Check sheet for the modelled part. Datum: model origin and axes. Units: mm. A direction names the side the tool comes from. Give positions to 0.01 mm unless a question says otherwise; leave off trailing zeros. Write each loop counter-clockwise with the first axis right and the second up, starting at its lowest first coordinate (ties: lowest second). Pieces come first, ordered by that corner, then holes. Notation, with made-up numbers: (22, 85.25) -> (38, 85.25) arc R22 cw to (38, 116.25) -> close; hole circle Ø3 at (60.5, -7.5). An arc over 180 degrees is marked (long way). Use a Markdown table: item, result. Add a question column.
1. Cross-section at B-B (x = 12.2). Enter the section's corners in (y, z).
2. Cross-section at D-D (y = 10.25). Enter the section's corners in (x, z).
3. Release check for a two-part mould opening along X. For faces 5 (the cylindrical face through (14.7, 5.8, 24.7)), 6 (the cylindrical face through (4.075, 4.5, 28.278)), 7 (the flat face through (11, 6, 0)) record: released by +X, released by -X, zero draft, split by the parting line, or undercut.
4. Cross-section at C-C (y = 3). Enter the section's corners in (x, z).
5. Cross-section at A-A (x = -2.4). Enter the section's corners in (y, z), then the cut area to 3 significant figures.
6. Scan lines: probe 1 along Y at (x, z) = (5.9, 27.35); probe 2 along Y at (x, z) = (-2.4, 16.65); probe 3 along X at (y, z) = (5.9, 17.4). Record each from-to range of solid material in increasing order. Write a range as [from, to].
7. Set-up check for faces 1 (the flat face through (22.5, 6, 21)), 2 (the flat face through (0, 6, 8)), 3 (the flat face through (24.8, 7.3, 15.9)), 4 (the cylindrical face through (0, 6, 25)): record each of +Z, -Z, +X, -X, +Y, -Y from which the full face is reachable in a straight line by a thin tool's end or side.
8. Gauge pin test, flat ends, axial feed: P1, Ø2, axis at y = 6.5, z = 20, coming from the +X side; P2, Ø1.8, axis at x = 3, y = 7.5, coming from the +Z side; P3, Ø1.4, axis at x = -1.5, y = 5, coming from the +Z side. Record the tip position at first contact, or that the pin passes through.
from build123d import *

# Parameters (mm, degrees)
CYLINDER005_R             = 0.85
CYLINDER005_DEPTH         = 4
CYLINDER004_R             = 2.3
CYLINDER004_DEPTH         = 3.3
CYLINDER003_R             = 2.5
CYLINDER003_DEPTH         = 4
CYLINDER002_R             = 5.9
CYLINDER002_DEPTH         = 4
BOX003_W                  = 22.5
BOX003_H                  = 11.8
BOX003_DEPTH              = 22.7
BOX002_W                  = 4.3
BOX002_H                  = 1.3
BOX002_DEPTH              = 5
CYLINDER001_R             = 1
CYLINDER001_DEPTH         = 5
FUSION001_PLACEMENT_ANGLE = 180
BOX001_W                  = 4.3
BOX001_H                  = 1.3
BOX001_DEPTH              = 5
CYLINDER_R                = 1
CYLINDER_DEPTH            = 5
BOX_W                     = 31.9
BOX_H                     = 11.8
BOX_DEPTH                 = 2.5


with BuildPart() as cylinder005:
    # Cylinder005 → Cylinder005 (new body)
    with BuildSketch(Plane.XY.offset(-0.5)):
        Circle(CYLINDER005_R)
    extrude(amount=CYLINDER005_DEPTH)


with BuildPart() as rotor:
    # Cylinder004 → Cylinder004 (new body)
    with BuildSketch(Plane.XY.offset(-0.1)):
        Circle(CYLINDER004_R)
    extrude(amount=CYLINDER004_DEPTH)

    # Cut002: cut Cylinder005
    add(cylinder005.part, mode=Mode.SUBTRACT)


with BuildPart() as rotor_1:
    # Cut002 placement: moved
    add(rotor.part.moved(Location((5.9, 5.9, 26.7))))


with BuildPart() as cylinder003:
    # Cylinder003 → Cylinder003 (new body)
    with BuildSketch(Plane(origin=(6.3, 0, 0), x_dir=(1, 0, 0), z_dir=(0, 0, 1))):
        Circle(CYLINDER003_R)
    extrude(amount=CYLINDER003_DEPTH)


with BuildPart() as soporte_con_rotor:
    # Cylinder002 → Cylinder002 (new body)
    with BuildSketch(Plane.XY):
        Circle(CYLINDER002_R)
    extrude(amount=CYLINDER002_DEPTH)

    # Fusion002: union Cylinder003
    add(cylinder003.part)


with BuildPart() as soporte_con_rotor_1:
    # Fusion002 placement: moved
    add(soporte_con_rotor.part.moved(Location((5.9, 5.9, 22.7))))

    # Fusion004: union rotor
    add(rotor_1.part)


with BuildPart() as base:
    # Box003 → Box003 (new body)
    with BuildSketch(Plane.XY):
        with Locations((11.25, 5.9)):
            Rectangle(BOX003_W, BOX003_H)
    extrude(amount=BOX003_DEPTH)


with BuildPart() as taladro_cubo001:
    # Box002 → Box002 (new body)
    with BuildSketch(Plane(origin=(0, -0.65, 0), x_dir=(1, 0, 0), z_dir=(0, 0, 1))):
        with Locations((2.15, 0.65)):
            Rectangle(BOX002_W, BOX002_H)
    extrude(amount=BOX002_DEPTH)


with BuildPart() as fusion001:
    # Cylinder001 → Cylinder001 (new body)
    with BuildSketch(Plane.XY):
        Circle(CYLINDER001_R)
    extrude(amount=CYLINDER001_DEPTH)

    # Fusion001: union taladro-cubo001
    add(taladro_cubo001.part)


with BuildPart() as fusion001_1:
    # Fusion001 placement: moved
    add(fusion001.part.moved(Location((2.3, 5.9, -1))).rotate(Axis((2.3, 5.9, -1), (0, 0, 1)), FUSION001_PLACEMENT_ANGLE))


with BuildPart() as taladro_cubo:
    # Box001 → Box001 (new body)
    with BuildSketch(Plane(origin=(0, -0.65, 0), x_dir=(1, 0, 0), z_dir=(0, 0, 1))):
        with Locations((2.15, 0.65)):
            Rectangle(BOX001_W, BOX001_H)
    extrude(amount=BOX001_DEPTH)


with BuildPart() as fusion:
    # Cylinder → Cylinder (new body)
    with BuildSketch(Plane.XY):
        Circle(CYLINDER_R)
    extrude(amount=CYLINDER_DEPTH)

    # Fusion: union taladro-cubo
    add(taladro_cubo.part)


with BuildPart() as fusion_1:
    # Fusion placement: moved
    add(fusion.part.moved(Location((29.6, 5.9, -1))))


with BuildPart() as fusion005:
    # Box → Box (new body)
    with BuildSketch(Plane.XY):
        with Locations((15.95, 5.9)):
            Rectangle(BOX_W, BOX_H)
    extrude(amount=BOX_DEPTH)

    # Cut: cut Fusion
    add(fusion_1.part, mode=Mode.SUBTRACT)

    # Cut001: cut Fusion001
    add(fusion001_1.part, mode=Mode.SUBTRACT)


with BuildPart() as fusion005_1:
    # Cut001 placement: moved
    add(fusion005.part.moved(Location((-4.7, 0, 15.9))))

    # Fusion003: union base
    add(base.part)

    # Fusion005: union soporte-con-rotor
    add(soporte_con_rotor_1.part)


solid = fusion005_1.part
Worked answers:
| question | item | result |
|---|---|---|
| 1 | outline | (0, 0) -> (11.8, 0) -> (11.8, 22.7) -> (8.4, 22.7) -> (8.4, 26.7) -> (3.4, 26.7) -> (3.4, 22.7) -> (0, 22.7) -> close |
| 2 | outline | (-4.7, 15.9) -> (0, 15.9) -> (0, 0) -> (22.5, 0) -> (22.5, 15.9) -> (27.2, 15.9) -> (27.2, 18.4) -> (22.5, 18.4) -> (22.5, 22.7) -> (9.89, 22.7) -> (9.89, 26.7) -> (1.91, 26.7) -> (1.91, 22.7) -> (0, 22.7) -> (0, 18.4) -> (-4.7, 18.4) -> close |
| 3 | face 5 | undercut |
| 3 | face 6 | split by the parting line |
| 3 | face 7 | zero draft |
| 4 | outline | (-4.7, 15.9) -> (0, 15.9) -> (0, 0) -> (22.5, 0) -> (22.5, 15.9) -> (27.2, 15.9) -> (27.2, 18.4) -> (22.5, 18.4) -> (22.5, 22.7) -> (11.04, 22.7) -> (11.04, 26.7) -> (0.76, 26.7) -> (0.76, 22.7) -> (0, 22.7) -> (0, 18.4) -> (-4.7, 18.4) -> close |
| 5 | outline | (0, 15.9) -> (4.9, 15.9) -> (4.9, 18.4) -> (0, 18.4) -> close; (6.9, 15.9) -> (11.8, 15.9) -> (11.8, 18.4) -> (6.9, 18.4) -> close |
| 5 | area | 24.5 mm² |
| 6 | probe 1 | y = [3.6, 5.05], [6.75, 8.2] |
| 6 | probe 2 | y = [0, 4.9], [6.9, 11.8] |
| 6 | probe 3 | x = [-1.4, 23.9] |
| 7 | face 1 | +Z, +X, +Y, -Y |
| 7 | face 2 | -Z, -X, +Y, -Y |
| 7 | face 3 | -Z, +X, +Y, -Y |
| 7 | face 4 | +Z |
| 8 | P1 | stops at x = 22.5 |
| 8 | P2 | stops at z = 26.7 |
| 8 | P3 | stops at z = 18.4 |
